Verification items for the finished model (mm, model axes). A direction names the side the tool comes from. Coordinates: 2 decimals unless noted, no trailing zeros. Loops run counter-clockwise (first coordinate to the right, second up) from the corner with the lowest first, then second, coordinate; pieces in that order, holes last. Notation, with made-up numbers: (-34.75, -27.75) - (22.25, -27.75) arc R7 ccw to (22.25, -17.75) - close; hole circle Ø1 at (-18.5, 36.5). An arc over 180 degrees is marked (long way). One line per item, written item: value. Start each with the question number.
(1) Section check B-B (x = 28). Record the boundary of the cut face in (y, z).
(2) Section check A-A (z = 1.7). Record the boundary of the cut face in (x, y).
(3) Thickness scan on probe 1 along Y at (x, z) = (23.5, 1.85); probe 2 along X at (y, z) = (-13.5, 2.15); probe 3 along X at (y, z) = (-6, 2.4). Record the ranges inside material, lowest first. Write a range as [from, to].
(4) Set-up check for faces 1 (the face through (-1, -10, 0)), 2 (the face through (18.5, -23, 1)), 3 (the face through (-39, -5, 1)), 4 (the face through (-35.5, 6, 1)), 5 (the face through (35.5, 6, 1)): record each of +Z, -Z, +X, -X, +Y, -Y from which the full face is reachable in a straight line by a thin tool's end or side.
(5) Gauge pin test, flat ends, axial feed: P1, Ø0.9, axis at x = -39.5, z = 1.5, coming from the +Y side; P2, Ø1.5, axis at y = -26, z = 1, coming from the +X side; P3, Ø0.8, axis at y = 6.5, z = 1.5, coming from the +X side. Record the tip position at first contact, or that the pin passes through.
(6) Section check C-C (y = -16.5). Record the boundary of the cut face in (x, z), plus the area to 3 significant figures.
```python
from build123d import *

# Parameters (mm, degrees)
ESBO_O1_W                = 71
ESBO_O1_H                = 15
ESBO_O1_W_2              = 20
ESBO_O1_H_2              = 30
ESBO_O1_W_3              = 6
ESBO_O1_H_3              = 10
RESSALTO_EXTRUS_O1_DEPTH = 3
FILETE1_R                = 5


with BuildPart() as part:
    # Esboço1 → Ressalto-extrusão1 (new body)
    with BuildSketch(Plane.XY):
        Rectangle(ESBO_O1_W, ESBO_O1_H)
        with Locations((8.5, -22.5)):
            Rectangle(ESBO_O1_W_2, ESBO_O1_H_2)
        with Locations((38.5, 0)):
            Rectangle(ESBO_O1_W_3, ESBO_O1_H_3)
        with Locations((-38.5, 0)):
            Rectangle(ESBO_O1_W_3, ESBO_O1_H_3)
    extrude(amount=RESSALTO_EXTRUS_O1_DEPTH)

    # Filete1
    filete1_edges = [part.edges().sort_by_distance(p)[0] for p in [
        (18.5, -7.5, 1.5),
        (18.5, -37.5, 1.5),
        (-1.5, -37.5, 1.5),
        (-1.5, -7.5, 1.5),
    ]]
    fillet(filete1_edges, radius=FILETE1_R)


solid = part.part
```
Responses:
1. outline: (-7.5, 0) - (7.5, 0) - (7.5, 3) - (-7.5, 3) - close
2. outline: (-41.5, -5) - (-35.5, -5) - (-35.5, -7.5) - (-6.5, -7.5) arc R5 cw to (-1.5, -12.5) - (-1.5, -32.5) arc R5 ccw to (3.5, -37.5) - (13.5, -37.5) arc R5 ccw to (18.5, -32.5) - (18.5, -12.5) arc R5 cw to (23.5, -7.5) - (35.5, -7.5) - (35.5, -5) - (41.5, -5) - (41.5, 5) - (35.5, 5) - (35.5, 7.5) - (-35.5, 7.5) - (-35.5, 5) - (-41.5, 5) - close
3. probe 1: y = [-7.5, 7.5]
3. probe 2: x = [-1.5, 18.5]
3. probe 3: x = [-35.5, 35.5]
4. face 1: -Z, +X, -X, +Y, -Y
4. face 2: +Z, -Z, +X, -Y
4. face 3: +Z, -Z, -X, -Y
4. face 4: +Z, -Z, -X, +Y
4. face 5: +Z, -Z, +X, +Y
5. P1: stops at y = 5
5. P2: stops at x = 18.5
5. P3: stops at x = 35.5
6. outline: (-1.5, 0) - (18.5, 0) - (18.5, 3) - (-1.5, 3) - close
6. area: 60.0 mm²
